Model file for the job. Use its own axes, mm. A direction names the side the tool comes from. Give positions to 0.01 mm unless a question says otherwise; leave off trailing zeros. Write each loop counter-clockwise with the first axis right and the second up, starting at its lowest first coordinate (ties: lowest second). Pieces come first, ordered by that corner, then holes. Notation, with made-up numbers: (9.25, -38) - (28.25, -38) arc R18 ccw to (28.25, -13) - close; hole circle Ø5 at (42.5, -27.75). An arc over 180 degrees is marked (long way). One line per item, written item: value. Start each with the question number.
(1) Cut at C-C, the plane y = 13. List the corners of the cut face in (x, z), and give its area (3 significant figures).
(2) Cut at A-A, the plane x = -10.75. List the corners of the cut face in (y, z).
(3) Mould opens along Y. For faces 3 (the face through (1.972, 6.974, 110.831)), 4 (the face through (4, -2, 111)), 5 (the face through (-5, -20, 111)) say: pulls with the +Y half, pulls with the -Y half, needs draft (parallel to the pull), parting line crosses it, or undercut.
(4) Drop flat-ended pins along their axis: P1, Ø3, axis at y = -9.5, z = 112, coming from the -X side; P2, Ø4.5, axis at y = 4.5, z = 68, coming from the -X side. Give the stop position or say it passes through.
(5) Probe L1, parallel to Z at x = 1.1, y = 7.5; L2, parallel to Z at x = -11, y = -10; L3, parallel to Y at x = 0.9, z = 192.5. List the from-to ranges inside material, lowest first.
(6) Cut at B-B, the plane z = 210. List the corners of the cut face in (x, y).
(7) 3-axis set-ups, long thin cutter, end or side, ignore diameter. For faces 1 (the face through (1.972, 6.974, 190.831)), 2 (the face through (-8, 0, 111)): which of +Z, -Z, +X, -X, +Y, -Y reach the whole face in a straight line?
Autodesk Inventor part; units mm, degrees
ref_plane "YZ Plane" through (0, 0, 0) normal (1, 0, 0) x (0, 1, 0)
ref_plane "XZ Plane" through (0, 0, 0) normal (0, 1, 0) x (-1, 0, 0)
ref_plane "XY Plane" through (0, 0, 0) normal (0, 0, 1) x (1, 0, 0)
sketch "Sketch1" plane through (0, 0, 0) normal (0, 0, 1) x (1, 0, 0)
  line L0 (0, 0) -> (0, 15)
  line L1 (0, 15) -> (4, 15)
  line L2 (4, 15) -> (4, -20)
  line L3 (4, -20) -> (-15, -20)
  line L4 (-15, -20) -> (-15, 0)
  line L5 (-15, 0) -> (0, 0)
  dimension "d0" = 15
  dimension "d1" = 4
  dimension "d2" = 35
extrude "Extrusion1" add sketch "Sketch1" along normal blind 225
sketch "Sketch2" plane through (4, -20, 0) normal (1, 0, 0) x (0, 0, -1)
  line L0 (0, 0) -> (0, 35)
  line L1 (0, 35) -> (-225, 35)
  line L2 (-225, 0) -> (-225, 35)
  line L3 (0, 0) -> (-225, 0)
  point P0 (0, 20)
  point P1 (-192.5, 27.5)
  point P2 (-112.5, 27.5)
  point P3 (-32.5, 27.5)
  point P4 (-112.5, 35)
  dimension "d5" = 80
  dimension "d6" = 80
  dimension "d7" = 7.5
hole "Hole1" at (4, 7.5, 192.5) at (4, 7.5, 112.5) at (4, 7.5, 32.5) direction (-1, 0, 0) diameter 3.5 end through all
chamfer "Chamfer1" distance 5 angle 45 2 edges at (-5.5, -20, 225) (-5.5, -20, 0)
sketch "Sketch3" plane through (-15, 0, 0) normal (-1, 0, 0) x (0, 0, 1)
  line L0 (5, -20) -> (220, -20)
  line L1 (225, -15) -> (220, -20)
  line L2 (225, 0) -> (225, -15)
  line L3 (5, -20) -> (0, -15)
  line L4 (0, 0) -> (0, -15)
  line L5 (0, 0) -> (225, 0)
  point P0 (32.5, -10)
  point P1 (112.5, -10)
  point P2 (192.5, -10)
  point P3 (112.5, -20)
  dimension "d18" = 80
  dimension "d19" = 80
  dimension "d20" = 10
hole "Hole2" at (-15, -10, 32.5) at (-15, -10, 112.5) at (-15, -10, 192.5) direction (1, 0, 0) diameter 2.8 depth 15
properties part number "Toolhead Dock Assembly" material "ABS Plastic"
Answers follow:
1. outline: (0, 0) - (4, 0) - (4, 225) - (0, 225) - close
1. area: 900 mm²
2. outline: (-20, 5) - (-15, 0) - (0, 0) - (0, 225) - (-15, 225) - (-20, 220) - close; hole circle Ø2.8 at (-10, 32.5); hole circle Ø2.8 at (-10, 112.5); hole circle Ø2.8 at (-10, 192.5)
3. face 3: undercut
3. face 4: needs draft
3. face 5: pulls with the -Y half
4. P1: stops at x = -15
4. P2: stops at x = 0
5. L1: z = 0 to 30.75, 34.25 to 110.75, 114.25 to 190.75, 194.25 to 225
5. L2: z = 0 to 31.1, 33.9 to 111.1, 113.9 to 191.1, 193.9 to 225
5. L3: y = -20 to 5.75, 9.25 to 15
6. outline: (-15, -20) - (4, -20) - (4, 15) - (0, 15) - (0, 0) - (-15, 0) - close
7. face 1: +X, -X
7. face 2: +Z, -Z, -X, +Y
